Design review of the part shown in the three views and the two pictorial views. Dimensions are in mm from the part's minimum x, y and z. A direction names the side the tool comes from. Round coordinates to 2 decimals unless told otherwise and drop trailing zeros. Order: outer loops, then holes, each group sorted by start corner. A loop starts at its lowest first (then second) coordinate and runs counter-clockwise, first axis right, second up.
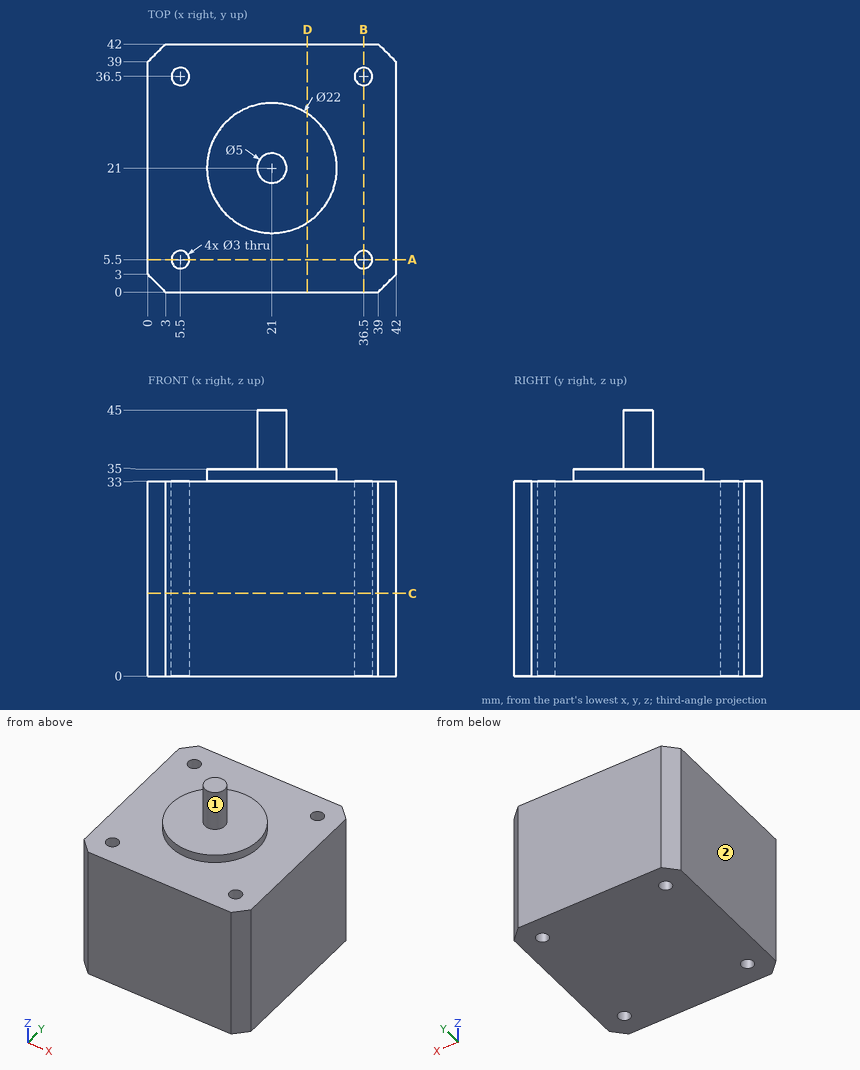
(1) Insertion check: pin 1 (6 mm diameter, centred on x = 8, y = 33, fed in from -Z); pin 2 (8 mm diameter, centred on x = 34.5, y = 15, fed in from +Z); pin 3 (1.5 mm diameter, centred on x = 37, y = 13.5, fed in from +Z). Each pin has a flat end and moves straight along its axis. Give the tip position at first contact, or say it passes through.
Data:
pin 1: stops at z = 0
pin 2: stops at z = 35
pin 3: stops at z = 33
(2) Consider section C-C (z = 14). Write out the cut boundary in (x, y), and give its area (3 significant figures).
Data:
outline: (0, 3) - (3, 0) - (39, 0) - (42, 3) - (42, 39) - (39, 42) - (3, 42) - (0, 39) - close; hole circle Ø3 at (5.5, 5.5); hole circle Ø3 at (5.5, 36.5); hole circle Ø3 at (36.5, 5.5); hole circle Ø3 at (36.5, 36.5)
area: 1,720 mm2
(3) For the marked faces 1 and 2, list the 3-axis set-ups (+Z, -Z, +X, -X, +Y, -Y) from which the entire face can be reached by the end or side of a thin tool; tool diameter is ignored.
Data:
face 1: +Z
face 2: +Z, -Z, -X, +Y, -Y
(4) Consider section A-A (y = 5.5). Write out the cut boundary in (x, z), and give its area (3 significant figures).
Data:
outline: (0, 0) - (4, 0) - (4, 33) - (0, 33) - close; (7, 0) - (35, 0) - (35, 33) - (7, 33) - close; (38, 0) - (42, 0) - (42, 33) - (38, 33) - close
area: 1,190 mm2
(5) Consider section D-D (x = 27). Write out the cut boundary in (y, z).
Data:
outline: (0, 0) - (42, 0) - (42, 33) - (30.22, 33) - (30.22, 35) - (11.78, 35) - (11.78, 33) - (0, 33) - close
(6) To check wall thickness, follow probe 1 along Y at (x, z) = (36.5, 18.5); probe 2 along Y at (x, z) = (5, 7); probe 3 along Z at (x, y) = (14, 16.5). State the ranges of each line that lie inside material, in increasing order.
Data:
probe 1: y = 0 to 4, 7 to 35, 38 to 42
probe 2: y = 0 to 4.09, 6.91 to 35.09, 37.91 to 42
probe 3: z = 0 to 35
